Verification items for this drawing (mm, ordinates from the low corner). A direction names the side the tool comes from. Coordinates: 2 decimals unless noted, no trailing zeros. Order: outer loops, then holes, each group sorted by start corner. A loop starts at its lowest first (then second) coordinate and runs counter-clockwise, first axis right, second up. Notation, with made-up numbers: M 83.25,46 L 92.25,46 A8 cw 92.25,55 Z; hole C 2,8 d11. An arc over 180 degrees is marked long. Return JSON: item names as keys, results as strings. Group by question number.
1. Set-up check for the marked faces 1 and 2: record each of +Z, -Z, +X, -X, +Y, -Y from which the full face is reachable in a straight line by a thin tool's end or side.
2. Section check A-A, the plane y = 35. Record the cut outline in (x, z), plus the area to 3 significant figures.
3. Material ranges on line 1 along Y through (x, z) = (16.5, 35); line 2 along Y through (x, z) = (29.5, 61.5), recorded low to high.
4. Gauge pin test, flat ends, axial feed: pin 1 (5 mm diameter, centred on x = 36, y = 10, fed in from -Z); pin 2 (12 mm diameter, centred on x = 13.5, y = 62.5, fed in from +Z); pin 3 (1.5 mm diameter, centred on x = 81, y = 17, fed in from -Z); pin 4 (4 mm diameter, centred on y = 35.5, z = 34, fed in from -X). Record the tip position at first contact, or that the pin passes through.
5. Section check B-B, the plane z = 43. Record the cut outline in (x, y), plus the area to 3 significant figures.
6. Section check C-C, the plane x = 37.5. Record the cut outline in (y, z), plus the area to 3 significant figures.
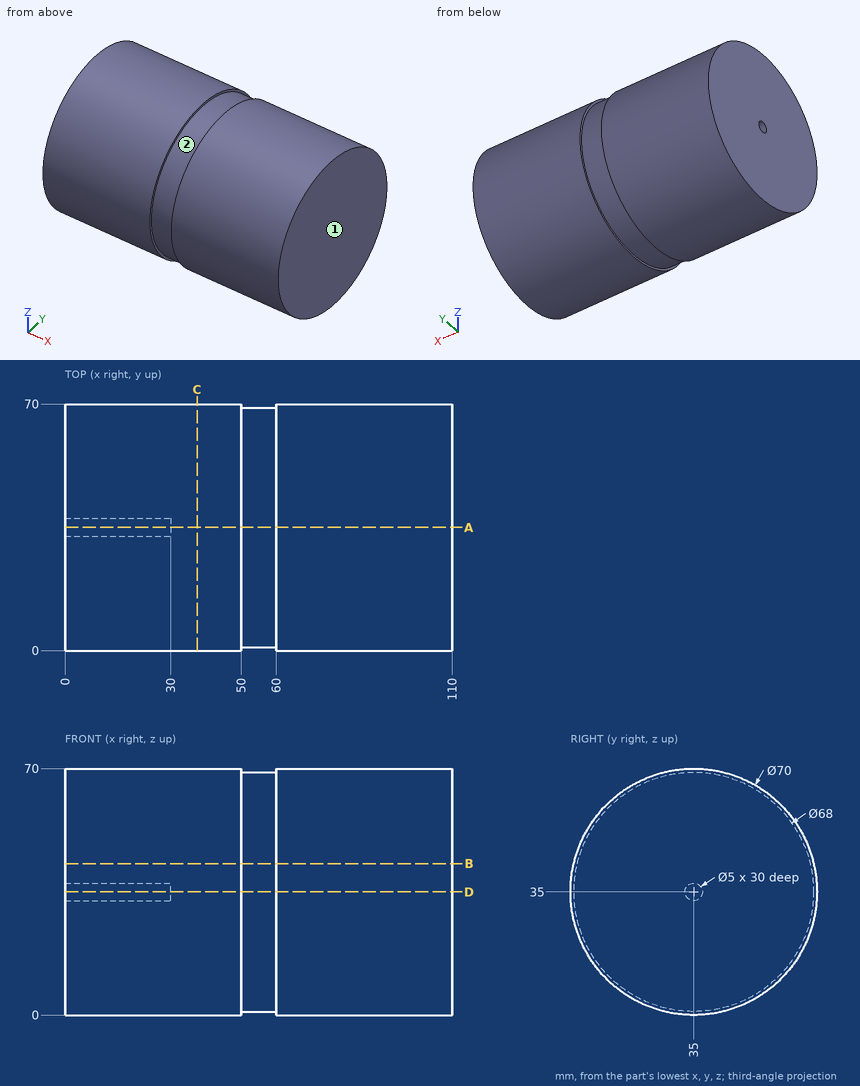
Answers follow:
{
 "1": {"face 1": "+Z, -Z, +X, +Y, -Y", "face 2": "none"},
 "2": {"outline": "M 0,0 L 50,0 L 50,1 L 60,1 L 60,0 L 110,0 L 110,70 L 60,70 L 60,69 L 50,69 L 50,70 L 0,70 L 0,37.5 L 30,37.5 L 30,32.5 L 0,32.5 Z", "area": "7,530 mm^2"},
 "3": {"line 1": "0 to 32.5, 37.5 to 70", "line 2": "12.14 to 57.86"},
 "4": {"pin 1": "z = 8.19", "pin 2": "z = 62.62", "pin 3": "z = 4.55", "pin 4": "x = 0"},
 "5": {"outline": "M 0,0.93 L 50,0.93 L 50,1.95 L 60,1.95 L 60,0.93 L 110,0.93 L 110,69.07 L 60,69.07 L 60,68.05 L 50,68.05 L 50,69.07 L 0,69.07 Z", "area": "7,480 mm^2"},
 "6": {"outline": "C 35,35 d70", "area": "3,850 mm^2"}
}
